Solid Edge part; units mm, degrees
sketch "Sketch1" plane through (0, 0, 0) normal (0, 0, 1) x (1, 0, 0)
  line L0 (-19.05, 0) -> (-9.525, -16.4978)
  line L1 (-9.525, -16.4978) -> (9.525, -16.4978)
  line L2 (9.525, -16.4978) -> (19.05, 0)
  line L3 (19.05, 0) -> (9.525, 16.4978)
  line L4 (9.525, 16.4978) -> (-9.525, 16.4978)
  line L5 (-9.525, 16.4978) -> (-19.05, 0)
  circle A0 centre (0, 0) radius 9.525
extrude "Protrusion1" add sketch "Sketch1" along normal blind 10.16
fillet "Round_1" radius 2.54 1 edges at (-9.525, 0, 10.16)
fillet "Round1" radius 0.635 1 edges at (-9.525, 0, 0)
chamfer "Chamfer_3" distance 1.27 angle 45 6 edges at (14.2875, 8.2489, 10.16) (14.2875, -8.2489, 10.16) (0, -16.4978, 10.16) (-14.2875, -8.2489, 10.16) (-14.2875, 8.2489, 10.16) (0, 16.4978, 10.16)
chamfer "Chamfer1" distance 1.27 angle 45 6 edges at (14.2875, -8.2489, 0) (0, -16.4978, 0) (-14.2875, -8.2489, 0) (-14.2875, 8.2489, 0) (0, 16.4978, 0) (14.2875, 8.2489, 0)
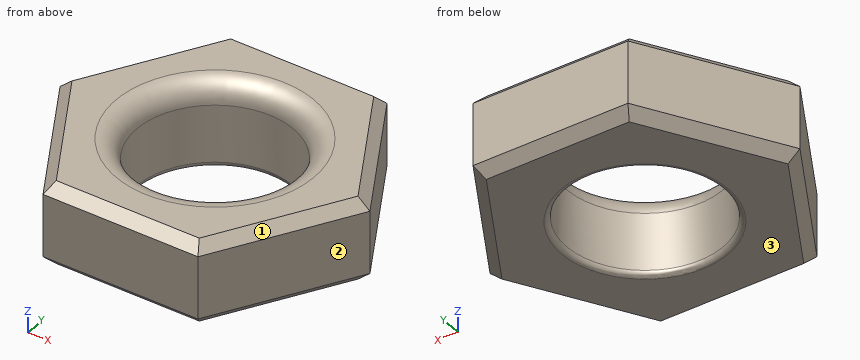
The listing builds one solid part. Answer for the finished solid, in the listing's coordinates (mm). Face numbers are marked on the shaded views. Round coordinates to 2 decimals unless told otherwise and drop trailing zeros. Order: outer loops, then holes, each group sorted by start corner. A loop starts at its lowest first (then second) coordinate and runs counter-clockwise, first axis right, second up. Notation, with made-up numbers: (-33.75, -24) -> (21.25, -24) arc R24 ccw to (21.25, 14) -> close; hole circle Ø10 at (41, 37). An arc over 180 degrees is marked (long way). Put each result on its own line as item: value.
Q1. Section B-B, the plane z = 4 is taken. Write down the section's boundary in (x, y) (3 decimals), and give its area (3 significant figures).
Results list:
outline: (-19.05, 0) -> (-9.525, -16.498) -> (9.525, -16.498) -> (19.05, 0) -> (9.525, 16.498) -> (-9.525, 16.498) -> close; hole circle Ø19.05 at (0, 0)
area: 658 mm^2
Q2. Section A-A, the plane x = 0 is taken. Write down the section's boundary in (y, z) (3 decimals).
Results list:
outline: (-16.498, 1.27) -> (-15.228, 0) -> (-10.16, 0) arc R0.635 ccw to (-9.525, 0.635) -> (-9.525, 7.62) arc R2.54 ccw to (-12.065, 10.16) -> (-15.228, 10.16) -> (-16.498, 8.89) -> close; (9.525, 0.635) arc R0.635 ccw to (10.16, 0) -> (15.228, 0) -> (16.498, 1.27) -> (16.498, 8.89) -> (15.228, 10.16) -> (12.065, 10.16) arc R2.54 ccw to (9.525, 7.62) -> close
Q3. Each of these flat-tipped pins is pushed along its axis until it touches: P1, Ø1, axis at x = 11.5, z = 4, coming from the -Y side; P2, Ø17, axis at x = 0, y = 0, coming from the -Z side; P3, Ø3, axis at y = -2, z = 1, coming from the -X side; P4, Ø5, axis at x = 15, z = 7, coming from the +Y side. Where does it stop, or does it pass through?
Results list:
P1: y = -13.94
P2: through
P3: x = -18.75
P4: y = 11.34
Q4. Consider line 1 along Y through (x, z) = (0, 4.5) (3 decimals); line 2 along X through (y, z) = (-4, 9); line 3 along X through (y, z) = (-0.5, 4). Determine where each line is inside the solid, lowest interval first.
Results list:
line 1: -16.498 to -9.525, 9.525 to 16.498
line 2: -16.61 to -9.09, 9.09 to 16.61
line 3: -18.76 to -9.51, 9.51 to 18.76
Q5. Determine the mould class of the marked faces 1, 2 and 3 for opening direction Z: pulls with the +Z half, pulls with the -Z half, needs draft (parallel to the pull), parting line crosses it, or undercut.
Results list:
face 1: pulls with the +Z half
face 2: needs draft
face 3: pulls with the -Z half
Q6. Section C-C, the plane x = 16 is taken. Write down the section's boundary in (y, z), and give its area (3 significant figures).
Results list:
outline: (-5.28, 1.27) -> (-2.74, 0) -> (2.74, 0) -> (5.28, 1.27) -> (5.28, 8.89) -> (2.74, 10.16) -> (-2.74, 10.16) -> (-5.28, 8.89) -> close
area: 101 mm^2
